from build123d import *

# Parameters (mm, degrees)
SKETCH1_R                       = 5
BOSS_EXTRUDE1_DEPTH             = 3.175
SKETCH6_W                       = 2.75
SKETCH6_H                       = 2.5
SKETCH6_H_2                     = 4
SKETCH6_W_2                     = 1.375
CUT_EXTRUDE4_DEPTH              = 109.300618445
CIRPATTERN1_COUNT               = 2
CIRPATTERN1_ANGLE               = 36
CIRPATTERN1_THE_OTHER_WAY_COUNT = 2
CIRPATTERN1_THE_OTHER_WAY_ANGLE = 36
F_3_0_3_DIAMETER_HOLE1_D        = 3


with BuildPart() as part:
    # Sketch1 → Boss-Extrude1 (new body)
    with BuildSketch(Plane(origin=(0, 0, 0), x_dir=(1, 0, 0), z_dir=(0, 1, 0))):
        with BuildLine():
            Line((-64.278760969, 0), (-6.749269902, -68.560977659))
            ThreePointArc((-6.749269902, -68.560977659), (0, -87.104444312), (6.749269902, -68.560977659))
            Line((6.749269902, -68.560977659), (64.278760969, 0))
            ThreePointArc((64.278760969, 0), (0, 23.395555688), (-64.278760969, 0))
        make_face()
        with Locations(Location((0, -76.604444312, 0), (0, 0, 270))):
            Circle(SKETCH1_R, mode=Mode.SUBTRACT)
        with BuildLine():
            Line((-49.832227183, -1.659470271), (-5, -55.08843808))
            Line((-5, -55.08843808), (-5, 13.256559466))
            ThreePointArc((-5, 13.256559466), (-28.412414016, 8.793065779), (-49.832227183, -1.659470271))
        make_face(mode=Mode.SUBTRACT)
        with BuildLine():
            Line((5, -55.08843808), (49.832227183, -1.659470271))
            ThreePointArc((49.832227183, -1.659470271), (28.412414016, 8.793065779), (5, 13.256559466))
            Line((5, 13.256559466), (5, -55.08843808))
        make_face(mode=Mode.SUBTRACT)
    extrude(amount=BOSS_EXTRUDE1_DEPTH)

    # Sketch6 → Cut-Extrude4 (cut, through all)
    with BuildSketch(Plane(origin=(0, 3.175, 0), x_dir=(1, 0, 0), z_dir=(0, 1, 0))):
        with Locations((0, 12.645555688)):
            Rectangle(SKETCH6_W, SKETCH6_H)
        with Locations((0, 15.895555688)):
            Rectangle(SKETCH6_W, SKETCH6_H_2)
        with Locations((-2.0625, 15.895555688)):
            Rectangle(SKETCH6_W_2, SKETCH6_H_2)
        with BuildLine():
            Line((-1.375, 23.386102116), (-1.375, 17.895555688))
            Line((-1.375, 17.895555688), (1.375, 17.895555688))
            Line((1.375, 17.895555688), (1.375, 23.386102116))
            ThreePointArc((1.375, 23.386102116), (0.687516249, 23.393192267), (0, 23.395555688))
            ThreePointArc((0, 23.395555688), (-0.687516249, 23.393192267), (-1.375, 23.386102116))
        make_face()
        with Locations((2.0625, 15.895555688)):
            Rectangle(SKETCH6_W_2, SKETCH6_H_2)
    cut_extrude4 = extrude(amount=-CUT_EXTRUDE4_DEPTH, mode=Mode.SUBTRACT)

    # CirPattern1: Cut-Extrude4 ×2 about axis
    cirpattern1_axis = Axis((0, 0, 76.604444312), (0, -1, 0))
    for i in range(1, CIRPATTERN1_COUNT):
        add(cut_extrude4.rotate(cirpattern1_axis, i * CIRPATTERN1_ANGLE / (CIRPATTERN1_COUNT - 1)), mode=Mode.SUBTRACT)

    # CirPattern1 the other way: Cut-Extrude4 ×2 about axis
    cirpattern1_the_other_way_axis = Axis((0, 0, 76.604444312), (0, 1, 0))
    for i in range(1, CIRPATTERN1_THE_OTHER_WAY_COUNT):
        add(cut_extrude4.rotate(cirpattern1_the_other_way_axis, i * CIRPATTERN1_THE_OTHER_WAY_ANGLE / (CIRPATTERN1_THE_OTHER_WAY_COUNT - 1)), mode=Mode.SUBTRACT)

    # Ø3.0 (3) Diameter Hole1 (through all)
    with Locations(Plane(origin=(0, 3.175, 0), x_dir=(1, 0, 0), z_dir=(0, 1, 0))):
        with Locations((0, -28.604444312), (-26.874184456, -36.798419304), (26.874184456, -36.798419304), (30.19139013, 13.470413235), (-29.356614466, 13.745924736)):
            Hole(F_3_0_3_DIAMETER_HOLE1_D / 2)


solid = part.part
Geometry check sheet. Reference: the model listing, model coordinates, mm. A direction names the side the tool comes from. Give positions to 0.01 mm unless a question says otherwise; leave off trailing zeros. Write each loop counter-clockwise with the first axis right and the second up, starting at its lowest first coordinate (ties: lowest second). Pieces come first, ordered by that corner, then holes. Notation, with made-up numbers: M 85.25,15 L 95.25,15 A26 ccw 95.25,43 Z; hole C 40.25,70 d10. An arc over 180 degrees is marked long. Answer as CSV lines item,"result". Start each with the question number.
Q1. Section check B-B, the plane z = 32.5. Record the cut outline in (x, y) (3 decimals), then the cut area to 3 significant figures.
Q2. Tool access check on faces 1 (the face through (0, 3.175, 23)), 2 (the face through (-56.58, 1.61, 3.41)). Record the directions out of +Z, -Z, +X, -X, +Y, -Y that give a thin tool (end or side, any length) a straight path to the whole face; none if there is none.
Q3. Section check C-C, the plane x = 44. Record the cut outline in (y, z) (3 decimals).
Q4. Go/stop test with flat-tipped pins: pin 1 (1 mm diameter, centred on x = 26, y = 2, fed in from +Z); pin 2 (1.6 mm diameter, centred on y = 2.5, z = -16.5, fed in from -X); pin 3 (1.6 mm diameter, centred on y = 2, z = 4.5, fed in from +X). Record where each tip stops, or that it passes through.
Q5. Release check for a two-part mould opening along Z. For faces 3 (the face through (0, 2, -11.396)), 4 (the face through (-2.75, 2, -16)), 5 (the face through (1.375, 2, -21)), 6 (the face through (0.195, 1.565, 27.117)) record: pulls with the +Z half, pulls with the -Z half, needs draft (parallel to the pull), parting line crosses it, or undercut.
Q6. Material ranges on L1, parallel to X at y = 1.5, z = -4.5; L2, parallel to X at y = 1.5, z = 49; L3, parallel to Z at x = 29, y = 2.4, recorded low to high.
Q7. Section check D-D, the plane y = 0.75. Give the number of separate pieces and of enclosed holes in the cut face, then the cut area to 3 significant figures.
Q8. Section check A-A, the plane x = 0. Record the cut outline in (y, z) (3 decimals).
Geometry says:
1,outline,"M -37.008,0 L -23.954,0 L -23.954,3.175 L -37.008,3.175 Z; M -5,0 L 5,0 L 5,3.175 L -5,3.175 Z; M 23.954,0 L 37.008,0 L 37.008,3.175 L 23.954,3.175 Z"
1,area,"115 mm^2"
2,face 1,"+Z, -Z, +X, -X, +Y"
2,face 2,"+Y, -Y"
3,outline,"M 0,-13.195 L 3.175,-13.195 L 3.175,-1.907 L 0,-1.907 Z; M 0,8.61 L 3.175,8.61 L 3.175,24.167 L 0,24.167 Z"
4,pin 1,"z = 46.21"
4,pin 2,"x = -38.47"
4,pin 3,"x = 61.17"
5,face 3,"pulls with the -Z half"
5,face 4,"undercut"
5,face 5,"needs draft"
5,face 6,"undercut"
6,L1,"-57.23 to -39.01, -5 to 5, 39.01 to 57.23"
6,L2,"-23.16 to -10.11, -5 to 5, 10.11 to 23.16"
6,L3,"-19.1 to -14.38, -12.56 to -8.6, 26.49 to 42.04"
7,separate pieces,"1"
7,enclosed holes,"8"
7,area,"3,740 mm^2"
8,outline,"M 0,-11.396 L 3.175,-11.396 L 3.175,27.104 L 0,27.104 Z; M 0,30.104 L 3.175,30.104 L 3.175,71.604 L 0,71.604 Z; M 0,81.604 L 3.175,81.604 L 3.175,87.104 L 0,87.104 Z"
